```python
from build123d import *

# Parameters (mm, degrees)
F0_W     = 476
F0_H     = 340
F0_W_2   = 456
F0_H_2   = 320
F1_DEPTH = 125
F2_DEPTH = 5
F3_R     = 15


with BuildPart() as f1:
    # F0 (on Top) → F1 (new body)
    with BuildSketch(Plane.XY):
        with Locations((-152.2744732499, 132.3741256595)):
            Rectangle(F0_W, F0_H)
        with Locations((-152.2744732499, 132.3741256595)):
            Rectangle(F0_W_2, F0_H_2, mode=Mode.SUBTRACT)
    extrude(amount=F1_DEPTH)

    # F0 (on Top) → F2 (join)
    with BuildSketch(Plane.XY):
        with Locations((-152.2744732499, 132.3741256595)):
            Rectangle(F0_W, F0_H)
        with Locations((-152.2744732499, 132.3741256595)):
            Rectangle(F0_W_2, F0_H_2, mode=Mode.SUBTRACT)
        with Locations((-152.2744732499, 132.3741256595)):
            Rectangle(F0_W_2, F0_H_2)
    extrude(amount=-F2_DEPTH)

    # F3
    f3_edges = [f1.edges().sort_by_distance(p)[0] for p in [
        (75.725527, 292.374126, 62.5),
        (-380.274473, 292.374126, 62.5),
        (75.725527, -27.625874, 62.5),
        (-380.274473, -27.625874, 62.5),
        (-152.274473, -27.625874, 0),
        (-380.274473, 132.374126, 0),
        (-152.274473, 292.374126, 0),
        (75.725527, 132.374126, 0),
    ]]
    fillet(f3_edges, radius=F3_R)


solid = f1.part
```
For this review, take the finished solid that the model builds, in its own axes (mm). A direction names the side the tool comes from. Coordinates: 2 decimals unless noted, no trailing zeros. Write each loop counter-clockwise with the first axis right and the second up, starting at its lowest first coordinate (ties: lowest second). Pieces come first, ordered by that corner, then holes. Notation, with made-up numbers: (55.25, 26.25) -> (106.25, 26.25) arc R22 cw to (106.25, 60.25) -> close; hole circle Ø10 at (86, 29.5). An arc over 180 degrees is marked (long way). Put each result on its own line as item: value.
Q1. Wall thickness on L1, parallel to Y at x = -140.5, z = 81.5; L2, parallel to X at y = 85.5, z = 79.5; L3, parallel to Z at x = -266.5, y = 268: over which ranges is each line inside the solid? List them lowest first.
From the geometry:
L1: y = -37.63 to -27.63, 292.37 to 302.37
L2: x = -390.27 to -380.27, 75.73 to 85.73
L3: z = -5 to 0
Q2. Take a section at C-C, the plane y = 261.5. State the section outline as (x, z) points.
From the geometry:
outline: (-390.27, -5) -> (85.73, -5) -> (85.73, 125) -> (75.73, 125) -> (75.73, 15) arc R15 cw to (60.73, 0) -> (-365.27, 0) arc R15 cw to (-380.27, 15) -> (-380.27, 125) -> (-390.27, 125) -> close
Q3. Take a section at A-A, the plane x = -256.5. State the section outline as (y, z) points.
From the geometry:
outline: (-37.63, -5) -> (302.37, -5) -> (302.37, 125) -> (292.37, 125) -> (292.37, 15) arc R15 cw to (277.37, 0) -> (-12.63, 0) arc R15 cw to (-27.63, 15) -> (-27.63, 125) -> (-37.63, 125) -> close
Q4. Take a section at B-B, the plane z = 60. State the section outline as (x, y) points, then the cut area to 3 significant figures.
From the geometry:
outline: (-390.27, -37.63) -> (85.73, -37.63) -> (85.73, 302.37) -> (-390.27, 302.37) -> close; hole (-380.27, -12.63) arc R15 ccw to (-365.27, -27.63) -> (60.73, -27.63) arc R15 ccw to (75.73, -12.63) -> (75.73, 277.37) arc R15 ccw to (60.73, 292.37) -> (-365.27, 292.37) arc R15 ccw to (-380.27, 277.37) -> close
area: 16,100 mm2
Q5. The part is to be moulded in two halves that separate along Y. For faces 1 (the flat face through (-156, 135, -5)), 2 (the flat face through (-156, -37.626, 61)), 3 (the flat face through (-156, 302.374, 61)), 4 (the cylindrical face through (-149.29, -23.12, 4.28)), say which applies: +Y half, -Y half, draft (parallel to the pull), parting line (faces both ways), or undercut.
From the geometry:
face 1: draft
face 2: -Y half
face 3: +Y half
face 4: undercut
Q6. Tool access review of faces 5 (the flat face through (-171, -31, 125)), 6 (the cylindrical face through (71.21, 288.1, 70.77)): name each direction out of +Z, -Z, +X, -X, +Y, -Y from which nothing blocks a thin tool from reaching the whole face with its end or side.
From the geometry:
face 5: +Z, +X, -X, +Y, -Y
face 6: +Z
